```python
from build123d import *

# Parameters (mm, degrees)
F1_DEPTH      = 127
F1_DEPTH_BACK = 25.4
F3_T          = -2.54


# Not quite as in the source:
# - a feature of the source that left no trace in its solid (it failed there, or was rolled back) is left out
# - a shell that OpenCascade refuses in one call is made with other operations: the cavity is built on its own and cut out


with BuildPart() as f1:
    # F0 (on Front) → F1 (new body, two sides)
    with BuildSketch(Plane.XZ) as f1_sk:
        with BuildLine():
            ThreePointArc((-12.7, 45.72), (0, 33.02), (12.7, 45.72))
            ThreePointArc((12.7, 45.72), (11.3033735945, 51.5099693768), (7.4206700182, 56.0264861364))
            ThreePointArc((7.4206700182, 56.0264861364), (-5.7899693768, 57.0233735945), (-12.7, 45.72))
        make_face()
        with BuildLine():
            ThreePointArc((7.4206700182, 56.0264861364), (11.3033735945, 51.5099693768), (12.7, 45.72))
            ThreePointArc((12.7, 45.72), (0, 33.02), (-12.7, 45.72))
            Line((-12.7, 45.72), (-12.7, 0))
            ThreePointArc((-12.7, 0), (0, 12.7), (12.7, 0))
            ThreePointArc((12.7, 0), (8.9802561211, -8.9802561211), (0, -12.7))
            Line((0, -12.7), (63.5, -12.7))
            ThreePointArc((63.5, -12.7), (51.4131812719, 3.8985655097), (70.9206700182, 10.3064861364))
            Line((70.9206700182, 10.3064861364), (7.4206700182, 56.0264861364))
        make_face()
        with BuildLine():
            ThreePointArc((76.2, 0), (74.8033735945, 5.7899693768), (70.9206700182, 10.3064861364))
            ThreePointArc((70.9206700182, 10.3064861364), (51.4131812719, 3.8985655097), (63.5, -12.7))
            ThreePointArc((63.5, -12.7), (72.4802561211, -8.9802561211), (76.2, 0))
        make_face()
        with BuildLine():
            ThreePointArc((12.7, 0), (0, 12.7), (-12.7, 0))
            ThreePointArc((-12.7, 0), (-8.9802561211, -8.9802561211), (0, -12.7))
            ThreePointArc((0, -12.7), (8.9802561211, -8.9802561211), (12.7, 0))
        make_face()
    extrude(amount=F1_DEPTH)
    extrude(f1_sk.sketch, amount=-F1_DEPTH_BACK)

    # F3: a shell. OpenCascade refuses it in one call, so the cavity is built on its own and cut out:
    # the body offset inwards by the wall thickness, plus a prism from it out through each open face.
    f3_core = offset(f1.part, amount=F3_T, mode=Mode.PRIVATE)
    f3_exits = [f3_core.faces().sort_by_distance(p)[0] for p in [
        (37.686536, -50.8, 31.105189),
    ]]
    add(f3_core, mode=Mode.SUBTRACT)
    extrude(f3_exits, amount=-F3_T, mode=Mode.SUBTRACT)


solid = f1.part
```
The listing builds one solid part. Answer for the finished solid, in the listing's coordinates (mm). A direction names the side the tool comes from. Round coordinates to 2 decimals unless told otherwise and drop trailing zeros. Order: outer loops, then holes, each group sorted by start corner. A loop starts at its lowest first (then second) coordinate and runs counter-clockwise, first axis right, second up. Notation, with made-up numbers: (51.25, -21) - (60.25, -21) arc R14 ccw to (60.25, -3) - close; hole circle Ø11 at (-28, 57). An arc over 180 degrees is marked (long way). Put each result on its own line as item: value. Start each with the question number.
(1) Find section A-A (y = -111.5). Give the vertices of the cut face in (x, z).
(2) Determine the mould class of faces 3 (the cylindrical face through (-4.493, -51.831, 54.833)), 4 (the cylindrical face through (-5.62, -51.87, 57.11)), 5 (the flat face through (31, -52, -12.7)) for opening direction X: released by +X, released by -X, zero draft, split by the parting line, or undercut.
(3) Find section C-C (x = 22). Give the vertices of the cut face in (y, z).
(4) Find section B-B (z = 29). Give the vertices of the cut face in (x, y).
(5) Given P1, Ø1, axis at x = 52.5, y = -102, coming from the +Z side; P2, Ø13.5, axis at y = -53.5, z = 14, coming from the +X side, each flat-ended and moving along its own axis, determine where each tip first touches the part or whether it passes through.
(6) Straight lines are drawn through the part: probe 1 along Y at (x, z) = (7.5, 45.5); probe 2 along Z at (x, y) = (0, -7); probe 3 along Z at (x, y) = (49, -80). For each, find the intervals that lie inside material, in ascending order. Write a range as from..to.
(7) For faces 1 (the flat face through (25, 22.86, 14)), 2 (the flat face through (-12.7, -52, 23)), determine the directions among +Z, -Z, +X, -X, +Y, -Y from which every point of the face is accessible in a straight line to the end or side of a thin tool.
Reply:
1. outline: (-12.7, 0) arc R12.7 ccw to (0, -12.7) - (63.5, -12.7) arc R12.7 ccw to (70.92, 10.31) - (69.44, 8.25) arc R10.16 cw to (63.5, -10.16) - (0, -10.16) arc R10.16 cw to (-10.16, 0) - (-10.16, 45.72) arc R10.16 cw to (5.94, 53.97) - (7.42, 56.03) arc R12.7 ccw to (-12.7, 45.72) - close
2. face 3: undercut
2. face 4: split by the parting line
2. face 5: zero draft
3. outline: (-127, -12.7) - (25.4, -12.7) - (25.4, 45.53) - (22.86, 45.53) - (22.86, -10.16) - (-124.46, -10.16) - (-124.46, 45.53) - (-127, 45.53) - close
4. outline: (-12.7, -127) - (44.96, -127) - (44.96, -124.46) - (-10.16, -124.46) - (-10.16, 22.86) - (44.96, 22.86) - (44.96, 25.4) - (-12.7, 25.4) - close
5. P1: z = -10.16
5. P2: x = 73.93
6. probe 1: -127..-124.46, 22.86..25.4
6. probe 2: -12.7..-10.16, 55.88..58.42
6. probe 3: -12.7..-10.16
7. face 1: none
7. face 2: +Z, -Z, -X, +Y, -Y
